from build123d import *

# Parameters (mm, degrees)
F1_DEPTH = 1.5
F0_W     = 64.5
F0_H     = 1
F0_W_2   = 1
F0_W_3   = 31.9007062912
F0_H_2   = 12.2398320138
F0_W_4   = 25.9428420663
F0_W_5   = 12.4608716816
F2_DEPTH = 0.5


with BuildPart() as f1:
    # F0 (on Top) → F1 (new body)
    with BuildSketch(Plane.XY):
        with BuildLine():
            Line((-63, -49), (63, -49))
            ThreePointArc((63, -49), (65.4748737342, -47.9748737342), (66.5, -45.5))
            Line((66.5, -45.5), (66.5, 45.5))
            ThreePointArc((66.5, 45.5), (65.4748737342, 47.9748737342), (63, 49))
            Line((63, 49), (-63, 49))
            ThreePointArc((-63, 49), (-65.4748737342, 47.9748737342), (-66.5, 45.5))
            Line((-66.5, 45.5), (-66.5, -45.5))
            ThreePointArc((-66.5, -45.5), (-65.4748737342, -47.9748737342), (-63, -49))
        make_face()
        with BuildLine():
            Line((0.5, 47.5), (63, 47.5))
            ThreePointArc((63, 47.5), (64.4142135624, 46.9142135624), (65, 45.5))
            Line((65, 45.5), (65, 35.2601679862))
            Line((65, 35.2601679862), (65, 34.2601679862))
            Line((65, 34.2601679862), (65, 18.6124684513))
            Line((65, 18.6124684513), (65, 17.6124684513))
            Line((65, 17.6124684513), (65, 7.1))
            Line((65, 7.1), (65, 6.1))
            Line((65, 6.1), (65, -26.4))
            Line((65, -26.4), (65, -27.4))
            Line((65, -27.4), (65, -37.9124684513))
            Line((65, -37.9124684513), (65, -38.9124684513))
            Line((65, -38.9124684513), (65, -45.5))
            ThreePointArc((65, -45.5), (64.4142135624, -46.9142135624), (63, -47.5))
            Line((63, -47.5), (0.5, -47.5))
            Line((0.5, -47.5), (-0.5, -47.5))
            Line((-0.5, -47.5), (-63, -47.5))
            ThreePointArc((-63, -47.5), (-64.4142135624, -46.9142135624), (-65, -45.5))
            Line((-65, -45.5), (-65, -38.9124684513))
            Line((-65, -38.9124684513), (-65, -37.9124684513))
            Line((-65, -37.9124684513), (-65, -27.4))
            Line((-65, -27.4), (-65, -26.4))
            Line((-65, -26.4), (-65, 6.1))
            Line((-65, 6.1), (-65, 7.1))
            Line((-65, 7.1), (-65, 17.6124684513))
            Line((-65, 17.6124684513), (-65, 18.6124684513))
            Line((-65, 18.6124684513), (-65, 34.2601679862))
            Line((-65, 34.2601679862), (-65, 35.2601679862))
            Line((-65, 35.2601679862), (-65, 45.5))
            ThreePointArc((-65, 45.5), (-64.4142135624, 46.9142135624), (-63, 47.5))
            Line((-63, 47.5), (-0.5, 47.5))
            Line((-0.5, 47.5), (0.5, 47.5))
        make_face(mode=Mode.SUBTRACT)
    extrude(amount=F1_DEPTH)

    # F0 (on Top) → F2 (join)
    with BuildSketch(Plane.XY):
        with Locations((-32.75, 34.7601679862)):
            Rectangle(F0_W, F0_H)
        with Locations((0, 34.7601679862)):
            Rectangle(F0_W_2, F0_H)
        with Locations((32.75, 34.7601679862)):
            Rectangle(F0_W, F0_H)
        with Locations((49.0496468544, 18.1124684513)):
            Rectangle(F0_W_3, F0_H)
        Polygon((0.5, -9.65), (0.5, 34.2601679862), (-0.5, 34.2601679862), (-0.5, -9.65), (-0.5, -10.65), (-0.5, -47.5), (0.5, -47.5), (0.5, -10.65), align=None)
        with Locations((0, 41.3800839931)):
            Rectangle(F0_W_2, F0_H_2)
        with Locations((-49.0496468544, 18.1124684513)):
            Rectangle(F0_W_3, F0_H)
        with Locations((52.0285789669, 6.6)):
            Rectangle(F0_W_4, F0_H)
        with Locations((52.0285789669, -26.9)):
            Rectangle(F0_W_4, F0_H)
        with Locations((6.7304358408, -10.15)):
            Rectangle(F0_W_5, F0_H)
        with Locations((-52.0285789669, 6.6)):
            Rectangle(F0_W_4, F0_H)
        with Locations((-6.7304358408, -10.15)):
            Rectangle(F0_W_5, F0_H)
        with Locations((-52.0285789669, -26.9)):
            Rectangle(F0_W_4, F0_H)
        with Locations((-49.0496468544, -38.4124684513)):
            Rectangle(F0_W_3, F0_H)
        with Locations((49.0496468544, -38.4124684513)):
            Rectangle(F0_W_3, F0_H)
    extrude(amount=F2_DEPTH)


solid = f1.part
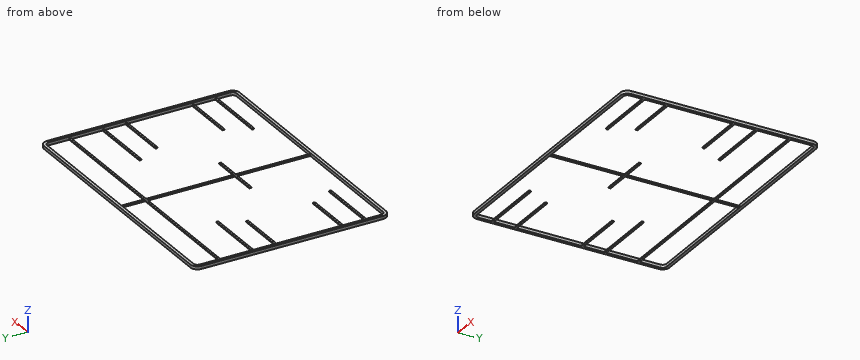
Could you check a few things on this model? Use its own coordinates, in mm. Round coordinates to 2 decimals unless told otherwise and drop trailing zeros. Write each loop counter-clockwise with the first axis right and the second up, starting at its lowest first coordinate (ties: lowest second). Pieces come first, ordered by that corner, then holes. Notation, with made-up numbers: (17, 63) - (69, 63) arc R25 ccw to (69, 102) - close; hole circle Ø3 at (-10.5, -32.75). An arc over 180 degrees is marked (long way). Use a Markdown table: item, result.
Q1. I want a section at D-D (y = 13.5). List the corners of the cut face in (x, z) for me, plus the area to 3 significant figures.
Output values:
| item | result |
|---|---|
| outline | (-66.5, 0) - (-65, 0) - (-65, 1.5) - (-66.5, 1.5) - close; (-0.5, 0) - (0.5, 0) - (0.5, 0.5) - (-0.5, 0.5) - close; (65, 0) - (66.5, 0) - (66.5, 1.5) - (65, 1.5) - close |
| area | 5.00 mm2 |
Q2. I want a section at A-A (x = -26). List the corners of the cut face in (y, z) for me.
Output values:
| item | result |
|---|---|
| outline | (-49, 0) - (-47.5, 0) - (-47.5, 1.5) - (-49, 1.5) - close; (34.26, 0) - (35.26, 0) - (35.26, 0.5) - (34.26, 0.5) - close; (47.5, 0) - (49, 0) - (49, 1.5) - (47.5, 1.5) - close |
Q3. Please list where these lines run through material, in increasing order: L1, parallel to X at y = 14, z = 0.35; L2, parallel to Y at x = -29, z = 0.25; L3, parallel to X at y = 43.5, z = 1.45.
Output values:
| item | result |
|---|---|
| L1 | -66.5 to -65, -0.5 to 0.5, 65 to 66.5 |
| L2 | -49 to -47.5, 34.26 to 35.26, 47.5 to 49 |
| L3 | -66.5 to -65, 65 to 66.5 |
Q4. I want a section at B-B (x = 41.5). List the corners of the cut face in (y, z) for me, plus the area to 3 significant figures.
Output values:
| item | result |
|---|---|
| outline | (-49, 0) - (-47.5, 0) - (-47.5, 1.5) - (-49, 1.5) - close; (-38.91, 0) - (-37.91, 0) - (-37.91, 0.5) - (-38.91, 0.5) - close; (-27.4, 0) - (-26.4, 0) - (-26.4, 0.5) - (-27.4, 0.5) - close; (6.1, 0) - (7.1, 0) - (7.1, 0.5) - (6.1, 0.5) - close; (17.61, 0) - (18.61, 0) - (18.61, 0.5) - (17.61, 0.5) - close; (34.26, 0) - (35.26, 0) - (35.26, 0.5) - (34.26, 0.5) - close; (47.5, 0) - (49, 0) - (49, 1.5) - (47.5, 1.5) - close |
| area | 7.00 mm2 |
Q5. I want a section at C-C (z = 0.9). List the corners of the cut face in (x, y) for me.
Output values:
| item | result |
|---|---|
| outline | (-66.5, -45.5) arc R3.5 ccw to (-63, -49) - (63, -49) arc R3.5 ccw to (66.5, -45.5) - (66.5, 45.5) arc R3.5 ccw to (63, 49) - (-63, 49) arc R3.5 ccw to (-66.5, 45.5) - close; hole (-65, -45.5) arc R2 ccw to (-63, -47.5) - (63, -47.5) arc R2 ccw to (65, -45.5) - (65, 45.5) arc R2 ccw to (63, 47.5) - (-63, 47.5) arc R2 ccw to (-65, 45.5) - close |
